Read the model definition and answer for the solid it produces. Units are mm, in the model's axes. A direction names the side the tool comes from. Give positions to 0.01 mm unless a question says otherwise; leave off trailing zeros. Write each loop counter-clockwise with the first axis right and the second up, starting at its lowest first coordinate (ties: lowest second). Pieces come first, ordered by that corner, then holes. Notation, with made-up numbers: (45.5, -31) - (89.5, -31) arc R20 ccw to (89.5, 0) - close; hole circle Ø11 at (57.25, -10.5). An arc over 180 degrees is marked (long way). Answer as a JSON object with one key per item and string values. Group by question number.
```python
from build123d import *

# Parameters (mm, degrees)
SKETCH_1_R          = 1.5
EXTRUDE_1_DEPTH     = 8
SKETCH_2_R          = 2
EXTRUDE_2_DEPTH     = 2.5
CUT_EXTRUDE_1_DEPTH = 1.5
FILLET_1_R          = 0.3
CHAMFER_1_SIZE      = 0.2


with BuildPart() as part:
    # 草图1 → 凸台-拉伸1 (new body)
    with BuildSketch(Plane.XY):
        Circle(SKETCH_1_R)
    extrude(amount=EXTRUDE_1_DEPTH)

    # 草图2 → 凸台-拉伸2 (add)
    with BuildSketch(Plane.XY.offset(8)):
        Circle(SKETCH_2_R)
    extrude(amount=EXTRUDE_2_DEPTH)

    # 草图3 → 切除-拉伸1 (cut)
    with BuildSketch(Plane.XY.offset(10.5)):
        Polygon((0, 1.480060872), (-1.281770315, 0.740030436), (-1.281770315, -0.740030436), (0, -1.480060872), (1.281770315, -0.740030436), (1.281770315, 0.740030436), align=None)
    extrude(amount=-CUT_EXTRUDE_1_DEPTH, mode=Mode.SUBTRACT)

    # 圆角1
    fillet_1_edges = [part.edges().sort_by_distance(p)[0] for p in [
        (-2, 0, 8),
        (-2, 0, 10.5),
    ]]
    fillet(fillet_1_edges, radius=FILLET_1_R)

    # 倒角1
    chamfer_1_edges = [part.edges().sort_by_distance(p)[0] for p in [
        (-1.5, 0, 0),
    ]]
    chamfer(chamfer_1_edges, length=CHAMFER_1_SIZE)


solid = part.part
```
1) Find section A-A, the plane y = 0. Write down the section's boundary in (x, z), and give its area (3 significant figures).
2) Find section B-B, the plane z = 2.25. Write down the section's boundary in (x, y).
3) Which of the six approach directions +Z, -Z, +X, -X, +Y, -Y give full straight-line access (tool end or side, diameter ignored) to faces 1 (the cylindrical face through (0, -2, 9)), 2 (the flat face through (1.282, 0, 10))?
4) Flat-ended cylindrical pins translate along their axes: pin 1 Ø1.2 at (y, z) = (0.5, 9.5) entering from -X; pin 2 Ø0.8 at (x, y) = (-0.5, 0.5) entering from +Z. Find the tip coordinate at first contact, or state that the pin passes through.
5) For a pull along X with two mould halves and no side action, classify faces 3 (the cylindrical face through (-1.5, 0.07, 4.05)), 4 (the flat face through (0, 0, 0)), 5 (the flat face through (0.65, 1.105, 9.76)), 6 (the flat face through (0, 0, 9)) as released by +X, released by -X, zero draft, split by the parting line, or undercut.
6) Find the intervals of material crossed by line 1 (Y direction, x = 0, z = 4); line 2 (Z direction, x = 1.7, y = 0.2); line 3 (Z direction, x = 1.1, y = -0.05), in increasing order. Write a range as [from, to].
Values follow:
{
 "1": {"outline": "(-2, 8.3) arc R0.3 ccw to (-1.7, 8) - (-1.5, 8) - (-1.5, 0.2) - (-1.3, 0) - (1.3, 0) - (1.5, 0.2) - (1.5, 8) - (1.7, 8) arc R0.3 ccw to (2, 8.3) - (2, 10.2) arc R0.3 ccw to (1.7, 10.5) - (1.28, 10.5) - (1.28, 9) - (-1.28, 9) - (-1.28, 10.5) - (-1.7, 10.5) arc R0.3 ccw to (-2, 10.2) - close", "area": "30.0 mm2"},
 "2": {"outline": "circle Ø3 at (0, 0)"},
 "3": {"face 1": "+Z, -Z", "face 2": "+Z"},
 "4": {"pin 1": "stops at x = -2", "pin 2": "stops at z = 9"},
 "5": {"face 3": "split by the parting line", "face 4": "zero draft", "face 5": "undercut", "face 6": "undercut"},
 "6": {"line 1": "y = [-1.5, 1.5]", "line 2": "z = [8, 10.5]", "line 3": "z = [0, 9]"}
}
